Source: CAD feature listing. Evaluate the final solid. Frame: model axes, mm. A direction names the side the tool comes from. Round coordinates to 2 decimals unless told otherwise and drop trailing zeros. Order: outer loops, then holes, each group sorted by start corner. A loop starts at its lowest first (then second) coordinate and runs counter-clockwise, first axis right, second up. Notation, with made-up numbers: (-3, 23) - (48, 23) arc R22 cw to (48, 44) - close; hole circle Ø3 at (-9.75, 33). An arc over 180 degrees is marked (long way). Put each result on its own line as item: value. Start each with the question number.
1) Mould query, pull axis Y, two halves, no side actions, for faces 3 (the face through (-9, 13, -22)), 4 (the face through (-17.11, -16.83, -18.55)), 5 (the face through (-11.435, -18.088, -18.549)), 6 (the face through (12.88, -14.95, -18.55)). Classes: +Y half, -Y half, draft (parallel to the pull), parting line (faces both ways), or undercut.
2) Section A-A on x = 8.5. Output: boundary loops of the cut face in (y, z).
3) Contact query for flat-ended pins moving along their axis: P1, Ø2.5, axis at x = -14.14, y = 14.14, coming from the -Z side; P2, Ø2, axis at x = 8.5, z = -16.5, coming from the +Y side. Output: stop coordinate, or through.
4) Access query for faces 1 (the face through (-9, 13, -15)), 2 (the face through (-18.752, -8.744, -18.549)). Directions: +Z, -Z, +X, -X, +Y, -Y. A direction counts if a zero-diameter tool reaches every point of the face in a straight line with its end or side. Return the directions, or none.
5) Line query: probe 1 along X at (y, z) = (-13, -20.25); probe 2 along X at (y, z) = (-17, -20.25); probe 3 along Y at (x, z) = (-9.5, -18). Output: solid intervals per line, ascending. Write a range as [from, to].
6) Section C-C on z = -16. Output: boundary loops of the cut face in (x, y).
7) Section D-D on y = -10.5. Output: boundary loops of the cut face in (x, z).
8) Section B-B on y = 3. Output: boundary loops of the cut face in (x, z), then the cut area to 3 significant figures.
```python
from build123d import *

# Parameters (mm, degrees)
CYLINDER804_R               = 20
CYLINDER804_DEPTH           = 7
BOX313_W                    = 1.4
BOX313_H                    = 60
BOX313_DEPTH                = 7
BOX313_PLACEMENT_ANGLE      = 5.7
BOX314_W                    = 1.4
BOX314_H                    = 60
BOX314_DEPTH                = 7
BOX314_PLACEMENT_ANGLE      = 3
CUT339_PLACEMENT_ANGLE      = 134.9
BOX311_W                    = 60
BOX311_H                    = 60
BOX311_DEPTH                = 7
BOX311_PLACEMENT_ANGLE      = 1
BOX312_W                    = 60
BOX312_H                    = 60
BOX312_DEPTH                = 7
BOX312_PLACEMENT_ANGLE      = 2
BOX310_W                    = 120
BOX310_H                    = 60
BOX310_DEPTH                = 7
TUBE084_R                   = 21.4
TUBE084_R_2                 = 20
TUBE084_DEPTH               = 7
BOX308_W                    = 60
BOX308_H                    = 60
BOX308_DEPTH                = 7
BOX308_PLACEMENT_ANGLE      = 20
BOX307_W                    = 60
BOX307_H                    = 60
BOX307_DEPTH                = 7
BOX307_PLACEMENT_ANGLE      = 20
BOX309_W                    = 120
BOX309_H                    = 60
BOX309_DEPTH                = 7
TUBE085_R                   = 21.4
TUBE085_R_2                 = 20
TUBE085_DEPTH               = 7
CUT335_PLACEMENT_ANGLE      = 135
CYLINDER811_R               = 1.5
CYLINDER811_DEPTH           = 20
CYLINDER811_PLACEMENT_ANGLE = 135
CYLINDER810_R               = 1.5
CYLINDER810_DEPTH           = 20
CYLINDER810_PLACEMENT_ANGLE = 45
BOX_W                       = 30.2
BOX_H                       = 30.2
BOX_DEPTH                   = 100
BOX_PLACEMENT_ANGLE         = 45
CYLINDER_R                  = 24
CYLINDER_DEPTH              = 7


with BuildPart() as obj1:
    # Cylinder804 → Cylinder804 (new body)
    with BuildSketch(Plane.XY.offset(-22)):
        Circle(CYLINDER804_R)
    extrude(amount=CYLINDER804_DEPTH)


with BuildPart() as krychle313:
    # Box313 → Box313 (new body)
    with BuildSketch(Plane.XY):
        with Locations((0.7, 30)):
            Rectangle(BOX313_W, BOX313_H)
    extrude(amount=BOX313_DEPTH)


with BuildPart() as krychle313_1:
    # Box313 placement: moved
    add(krychle313.part.moved(Location((0, 0, -22))).rotate(Axis((0, 0, -22), (0, 0, 1)), BOX313_PLACEMENT_ANGLE))


with BuildPart() as cut339:
    # Box314 → Box314 (new body)
    with BuildSketch(Plane.XY):
        with Locations((0.7, 30)):
            Rectangle(BOX314_W, BOX314_H)
    extrude(amount=BOX314_DEPTH)


with BuildPart() as cut339_1:
    # Box314 placement: moved
    add(cut339.part.moved(Location((0, 0, -22))).rotate(Axis((0, 0, -22), (0, 0, -1)), BOX314_PLACEMENT_ANGLE))

    # Compound720: union Krychle313
    add(krychle313_1.part)

    # Cut339: cut obj1
    add(obj1.part, mode=Mode.SUBTRACT)


with BuildPart() as cut339_2:
    # Cut339 placement: moved
    add(cut339_1.part.rotate(Axis((0, 0, 0), (0, 0, 1)), CUT339_PLACEMENT_ANGLE))


with BuildPart() as krychle311:
    # Box311 → Box311 (new body)
    with BuildSketch(Plane.XY):
        with Locations((30, 30)):
            Rectangle(BOX311_W, BOX311_H)
    extrude(amount=BOX311_DEPTH)


with BuildPart() as krychle311_1:
    # Box311 placement: moved
    add(krychle311.part.moved(Location((-59.990862, -1.047144, -22))).rotate(Axis((-59.990862, -1.047144, -22), (0, 0, 1)), BOX311_PLACEMENT_ANGLE))


with BuildPart() as compound719:
    # Box312 → Box312 (new body)
    with BuildSketch(Plane.XY):
        with Locations((30, 30)):
            Rectangle(BOX312_W, BOX312_H)
    extrude(amount=BOX312_DEPTH)


with BuildPart() as compound719_1:
    # Box312 placement: moved
    add(compound719.part.moved(Location((0, 0, -22))).rotate(Axis((0, 0, -22), (0, 0, -1)), BOX312_PLACEMENT_ANGLE))

    # Compound719: union Krychle311
    add(krychle311_1.part)


with BuildPart() as krychle310:
    # Box310 → Box310 (new body)
    with BuildSketch(Plane(origin=(-60, -60, -22), x_dir=(1, 0, 0), z_dir=(0, 0, 1))):
        with Locations((60, 30)):
            Rectangle(BOX310_W, BOX310_H)
    extrude(amount=BOX310_DEPTH)


with BuildPart() as cut338:
    # Tube084 → Tube084 (new body)
    with BuildSketch(Plane.XY.offset(-22)):
        Circle(TUBE084_R)
        Circle(TUBE084_R_2, mode=Mode.SUBTRACT)
    extrude(amount=TUBE084_DEPTH)

    # Cut337: cut Krychle310
    add(krychle310.part, mode=Mode.SUBTRACT)

    # Cut338: cut Compound719
    add(compound719_1.part, mode=Mode.SUBTRACT)


with BuildPart() as cut338_1:
    # Cut338 placement: moved
    add(cut338.part.moved(Location((0, 0, -7))))


with BuildPart() as krychle308:
    # Box308 → Box308 (new body)
    with BuildSketch(Plane.XY):
        with Locations((30, 30)):
            Rectangle(BOX308_W, BOX308_H)
    extrude(amount=BOX308_DEPTH)


with BuildPart() as krychle308_1:
    # Box308 placement: moved
    add(krychle308.part.moved(Location((-56.381557, -20.521209, -22))).rotate(Axis((-56.381557, -20.521209, -22), (0, 0, 1)), BOX308_PLACEMENT_ANGLE))


with BuildPart() as compound718:
    # Box307 → Box307 (new body)
    with BuildSketch(Plane.XY):
        with Locations((30, 30)):
            Rectangle(BOX307_W, BOX307_H)
    extrude(amount=BOX307_DEPTH)


with BuildPart() as compound718_1:
    # Box307 placement: moved
    add(compound718.part.moved(Location((0, 0, -22))).rotate(Axis((0, 0, -22), (0, 0, -1)), BOX307_PLACEMENT_ANGLE))

    # Compound718: union Krychle308
    add(krychle308_1.part)


with BuildPart() as krychle309:
    # Box309 → Box309 (new body)
    with BuildSketch(Plane(origin=(-60, -60, -22), x_dir=(1, 0, 0), z_dir=(0, 0, 1))):
        with Locations((60, 30)):
            Rectangle(BOX309_W, BOX309_H)
    extrude(amount=BOX309_DEPTH)


with BuildPart() as cut335:
    # Tube085 → Tube085 (new body)
    with BuildSketch(Plane.XY.offset(-22)):
        Circle(TUBE085_R)
        Circle(TUBE085_R_2, mode=Mode.SUBTRACT)
    extrude(amount=TUBE085_DEPTH)

    # Cut334: cut Krychle309
    add(krychle309.part, mode=Mode.SUBTRACT)

    # Cut336: cut Compound718
    add(compound718_1.part, mode=Mode.SUBTRACT)


with BuildPart() as cut335_1:
    # Cut336 placement: moved
    add(cut335.part.moved(Location((0, 0, -7))))

    # Cut335: cut Cut338
    add(cut338_1.part, mode=Mode.SUBTRACT)


with BuildPart() as cut335_2:
    # Cut335 placement: moved
    add(cut335_1.part.moved(Location((0, 0, 7))).rotate(Axis((0, 0, 7), (0, 0, 1)), CUT335_PLACEMENT_ANGLE))


with BuildPart() as obj2:
    # Cylinder811 → Cylinder811 (new body)
    with BuildSketch(Plane.XY):
        Circle(CYLINDER811_R)
    extrude(amount=CYLINDER811_DEPTH)


with BuildPart() as obj2_1:
    # Cylinder811 placement: moved
    add(obj2.part.moved(Location((-14.142136, 14.142136, -30))).rotate(Axis((-14.142136, 14.142136, -30), (0, 0, 1)), CYLINDER811_PLACEMENT_ANGLE))


with BuildPart() as compound721:
    # Cylinder810 → Cylinder810 (new body)
    with BuildSketch(Plane.XY):
        Circle(CYLINDER810_R)
    extrude(amount=CYLINDER810_DEPTH)


with BuildPart() as compound721_1:
    # Cylinder810 placement: moved
    add(compound721.part.moved(Location((14.142136, -14.142136, -30))).rotate(Axis((14.142136, -14.142136, -30), (0, 0, -1)), CYLINDER810_PLACEMENT_ANGLE))

    # Compound721: union obj2
    add(obj2_1.part)


with BuildPart() as krychle:
    # Box → Box (new body)
    with BuildSketch(Plane.XY):
        with Locations((15.1, 15.1)):
            Rectangle(BOX_W, BOX_H)
    extrude(amount=BOX_DEPTH)


with BuildPart() as krychle_1:
    # Box placement: moved
    add(krychle.part.moved(Location((0, -21.354625, -30))).rotate(Axis((0, -21.354625, -30), (0, 0, 1)), BOX_PLACEMENT_ANGLE))


with BuildPart() as cut348:
    # Cylinder → Cylinder (new body)
    with BuildSketch(Plane.XY.offset(-22)):
        Circle(CYLINDER_R)
    extrude(amount=CYLINDER_DEPTH)

    # Cut: cut Krychle
    add(krychle_1.part, mode=Mode.SUBTRACT)

    # Cut343: cut Compound721
    add(compound721_1.part, mode=Mode.SUBTRACT)

    # Cut347: cut Cut335
    add(cut335_2.part, mode=Mode.SUBTRACT)

    # Cut348: cut Cut339
    add(cut339_2.part, mode=Mode.SUBTRACT)


solid = cut348.part
```
Answer sheet:
1. face 3: draft
1. face 4: -Y half
1. face 5: undercut
1. face 6: undercut
2. outline: (-22.44, -22) - (-12.85, -22) - (-12.85, -15) - (-22.44, -15) - close; (12.85, -22) - (22.44, -22) - (22.44, -15) - (12.85, -15) - close
3. P1: through
3. P2: y = 22.8
4. face 1: +Z, +X, -X, +Y, -Y
4. face 2: +Z, -Z
5. probe 1: [-20.17, -17], [-15.2, -8.35], [8.35, 13.17], [15.11, 20.17]
5. probe 2: [-16.94, -15.78], [-13.96, -13], [-10.54, -4.35], [4.35, 16.94]
5. probe 3: [-22.04, -19.18], [-17.6, -11.85], [11.85, 22.04]
6. outline: (-19.39, -9.04) - (-18.13, -8.45) arc R20 ccw to (-14.63, -13.64) - (-15.65, -14.59) arc R21.4 cw to (-15.93, -14.29) - (-17.86, -16.03) arc R24 ccw to (-16.29, -17.63) - (-14.64, -15.61) arc R21.4 cw to (-14.87, -15.39) - (-13.89, -14.39) arc R20 ccw to (-8.45, -18.13) - (-9.04, -19.39) arc R21.4 cw to (-13.58, -16.54) - (-15.23, -18.55) arc R24 ccw (long way) to (-18.77, -14.96) - (-16.83, -13.22) arc R21.4 cw to start; hole (-21.35, 0) - (0, -21.35) - (21.35, 0) - (0, 21.35) - close; hole circle Ø3 at (-14.14, 14.14); hole circle Ø3 at (14.14, -14.14)
7. outline: (-21.58, -22) - (-18.65, -22) - (-18.65, -15) - (-21.58, -15) - close; (-17.02, -22) - (-10.85, -22) - (-10.85, -15) - (-17.02, -15) - close; (10.85, -22) - (21.58, -22) - (21.58, -15) - (10.85, -15) - close
8. outline: (-23.81, -22) - (-18.35, -22) - (-18.35, -15) - (-23.81, -15) - close; (18.35, -22) - (23.81, -22) - (23.81, -15) - (18.35, -15) - close
8. area: 76.4 mm^2
